Check sheet for the modelled part. Datum: model origin and axes. Units: mm. Face numbers are marked on the shaded views. A direction names the side the tool comes from. Give positions to 0.01 mm unless a question says otherwise; leave off trailing zeros. Write each loop counter-clockwise with the first axis right and the second up, starting at its lowest first coordinate (ties: lowest second). Pieces come first, ordered by that corner, then holes. Notation, with made-up numbers: M -29.5,-24.5 L 13.5,-24.5 A23 cw 13.5,-7.5 Z; hole C 33,84.5 d1. An arc over 180 degrees is marked long. Use CSV: the item, a comma, the result in double quotes. Start each with the question number.
1. Depth check by flat-ended pin: P1, Ø0.7, axis at x = 55.5, y = -24.5, coming from the -Z side; P2, Ø5, axis at x = 45, y = 3.5, coming from the -Z side; P3, Ø5, axis at y = 27.5, z = 34.5, coming from the -X side. Enter the tip coordinate at first touch or a pass-through.
2. Cross-section at A-A, the plane z = 3. Enter the section's corners in (x, y) (3 decimals).
3. Cross-section at B-B, the plane y = 10. Enter the section's corners in (x, z) (3 decimals), and give its area (3 significant figures).
4. Cross-section at C-C, the plane x = 98. Enter the section's corners in (y, z) (3 decimals), and give its area (3 significant figures).
5. Scan lines: line 1 (X direction, y = -23.5, z = 6.5) (3 decimals); line 2 (Z direction, x = -34, y = 41) (3 decimals); line 3 (Z direction, x = 72, y = 25.5) (3 decimals). Record each from-to range of solid material in increasing order.
6. Access from +Z, -Z, +X, -X, +Y, -Y to the whole of each face (thin tool, end or side, straight path). Record for the marked faces 1, 2, 3 and 4.
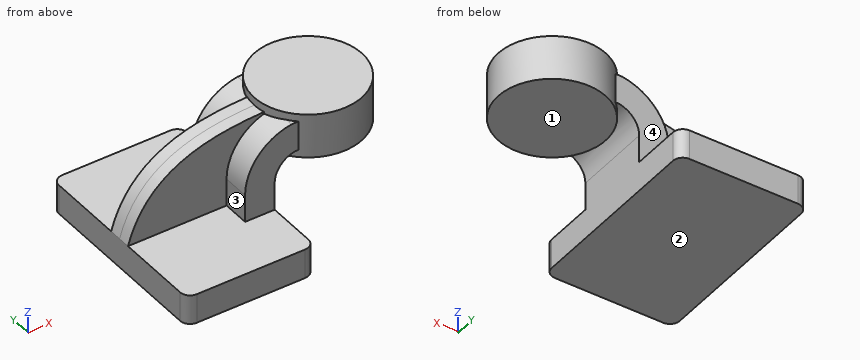
from build123d import *

# Parameters (mm, degrees)
F1_DEPTH = 63.5
F0_W     = 16.14231
F0_H     = 19.05
F2_DEPTH = 25.4
F3_DEPTH = 7.9375
F5_R     = 6.35


with BuildPart() as f1:
    # F0 (on Front) → F1 (new body, symmetric)
    with BuildSketch(Plane.XZ):
        Polygon((22.225, 9.525), (-41.275, 9.525), (-41.275, -9.525), (41.275, -9.525), (41.275, 9.525), align=None)
    extrude(amount=F1_DEPTH, both=True)

    # F0 (on Front) → F2 (join, symmetric)
    with BuildSketch(Plane.XZ):
        with BuildLine():
            Line((22.225, 27.245483), (22.225, 9.525))
            Line((22.225, 9.525), (41.275, 9.525))
            Line((41.275, 9.525), (41.275, 27.245483))
            ThreePointArc((41.275, 27.245483), (44.98148, 37.440715), (54.37015, 42.8752))
            Line((54.37015, 42.8752), (63.990081, 42.8752))
            Line((63.990081, 42.8752), (63.990081, 61.9252))
            add(Edge.make_bspline(
                [(52.118676, 61.806174), (56.173728, 61.882453), (60.147361, 61.905409), (63.990081, 61.9252)],
                knots=[105.880796, 105.880796, 105.880796, 105.880796, 117.586216, 117.586216, 117.586216, 117.586216], degree=3))
            ThreePointArc((52.118676, 61.806174), (30.735282, 50.093203), (22.225, 27.245483))
        make_face()
        with Locations((72.061236, 52.4002)):
            Rectangle(F0_W, F0_H)
    extrude(amount=F2_DEPTH, both=True)

    # F0 (on Front) → F3 (join, symmetric)
    with BuildSketch(Plane.XZ):
        with BuildLine():
            add(Edge.make_bspline(
                [(-41.275, 9.525), (-27.902543, 56.063321), (15.438907, 61.1162), (52.118676, 61.806174)],
                knots=[0, 0, 0, 0, 105.880796, 105.880796, 105.880796, 105.880796], degree=3))
            Line((-41.275, 9.525), (22.225, 9.525))
            Line((22.225, 9.525), (22.225, 27.245483))
            ThreePointArc((22.225, 27.245483), (30.735282, 50.093203), (52.118676, 61.806174))
        make_face()
    extrude(amount=F3_DEPTH, both=True)

    # F0 (on Front) → F4 (revolve)
    with BuildSketch(Plane.XZ):
        Polygon((80.132391, 66.675), (80.132391, 61.9252), (80.132391, 42.8752), (80.132391, 38.1), (114.790081, 38.1), (114.790081, 66.675), align=None)
    revolve(axis=Axis((80.132391, 0, 52.3875), (0, 0, 1)))

    # F5
    f5_edges = [f1.edges().sort_by_distance(p)[0] for p in [
        (41.275, 63.5, 0),
        (-41.275, 63.5, 0),
        (-41.275, -63.5, 0),
        (41.275, -63.5, 0),
    ]]
    fillet(f5_edges, radius=F5_R)


solid = f1.part
Worked answers:
1,P1,"stops at z = 38.1"
1,P2,"stops at z = 33.36"
1,P3,"stops at x = 22.73"
2,outline,"M -41.275,-57.15 A6.35 ccw -34.925,-63.5 L 34.925,-63.5 A6.35 ccw 41.275,-57.15 L 41.275,57.15 A6.35 ccw 34.925,63.5 L -34.925,63.5 A6.35 ccw -41.275,57.15 Z"
3,outline,"M -41.275,-9.525 L 41.275,-9.525 L 41.275,27.245 A15.875 cw 46.949,39.409 L 46.949,38.1 L 113.316,38.1 L 113.316,66.675 L 46.949,66.675 L 46.949,60.647 A34.925 ccw 22.225,27.245 L 22.225,9.525 L -41.275,9.525 Z"
3,area,"4,370 mm^2"
4,outline,"M -29.697,38.1 L 29.697,38.1 L 29.697,66.675 L -29.697,66.675 Z"
4,area,"1,700 mm^2"
5,line 1,"x = -41.275 to 41.275"
5,line 2,"z = -9.525 to 9.525"
5,line 3,"z = 38.1 to 66.675"
6,face 1,"-Z, +X, +Y, -Y"
6,face 2,"-Z, +X, -X, +Y, -Y"
6,face 3,"+Z, -X, -Y"
6,face 4,"+Z, -X, +Y"
